```python
from build123d import *

# Parameters (mm, degrees)
SKETCH101_W          = 122
SKETCH101_H          = 70.3
SKETCH101_R          = 1.75
SKETCH101_R_2        = 1.55
SKETCH101_W_2        = 52.2
SKETCH101_H_2        = 52.2
PAD033_DEPTH         = 4
FILLET008_R          = 2
SKETCH102_W          = 2
SKETCH102_H          = 2.1
POCKET051_DEPTH      = 35.151
POCKET051_DEPTH_BACK = 35.151
SKETCH103_R          = 3
POCKET039_DEPTH      = 2.001
SKETCH104_W          = 4.202
SKETCH104_H          = 4.8
PAD035_DEPTH         = 10
CHAMFER004_SIZE2     = 9.99
CHAMFER004_SIZE      = 1.99


with BuildPart() as part:
    # Sketch101 → Pad033 (new body)
    with BuildSketch(Plane.XY):
        with Locations((31, 0)):
            Rectangle(SKETCH101_W, SKETCH101_H)
        with Locations((0, 31.75)):
            Circle(SKETCH101_R, mode=Mode.SUBTRACT)
        with Locations((-14, 30.5)):
            Circle(SKETCH101_R_2, mode=Mode.SUBTRACT)
        with Locations((60, 31.75)):
            Circle(SKETCH101_R, mode=Mode.SUBTRACT)
        with Locations((46, 30.5)):
            Circle(SKETCH101_R_2, mode=Mode.SUBTRACT)
        with Locations((60, -31.75)):
            Circle(SKETCH101_R, mode=Mode.SUBTRACT)
        with Locations((0, -31.75)):
            Circle(SKETCH101_R, mode=Mode.SUBTRACT)
        Rectangle(SKETCH101_W_2, SKETCH101_H_2, mode=Mode.SUBTRACT)
        with Locations((60, 0)):
            Rectangle(SKETCH101_W_2, SKETCH101_H_2, mode=Mode.SUBTRACT)
    extrude(amount=PAD033_DEPTH)

    # Fillet008
    fillet008_edges = [part.edges().sort_by_distance(p)[0] for p in [
        (31, 35.15, 4),
        (31, -35.15, 4),
    ]]
    fillet(fillet008_edges, radius=FILLET008_R)

    # Sketch102 → Pocket051 (cut, two sides)
    with BuildSketch(Plane.XZ) as pocket051_sk:
        with Locations((-29, 2.95)):
            Rectangle(SKETCH102_W, SKETCH102_H)
        with Locations((91, 1.05)):
            Rectangle(SKETCH102_W, SKETCH102_H)
    extrude(amount=-POCKET051_DEPTH, mode=Mode.SUBTRACT)
    extrude(pocket051_sk.sketch, amount=POCKET051_DEPTH_BACK, mode=Mode.SUBTRACT)

    # Sketch103 → Pocket039 (cut, through all)
    with BuildSketch(Plane.XY.offset(2)):
        with Locations((0, 31.75)):
            Circle(SKETCH103_R)
        with Locations((60, 31.75)):
            Circle(SKETCH103_R)
        with Locations((60, -31.75)):
            Circle(SKETCH103_R)
        with Locations((0, -31.75)):
            Circle(SKETCH103_R)
    extrude(amount=POCKET039_DEPTH, mode=Mode.SUBTRACT)

    # Sketch104 → Pad035 (join)
    with BuildSketch(Plane.XY):
        with Locations((-25.899, 30.75)):
            Rectangle(SKETCH104_W, SKETCH104_H)
        with Locations((-25.899, -30.75)):
            Rectangle(SKETCH104_W, SKETCH104_H)
    extrude(amount=-PAD035_DEPTH)

    # Chamfer004
    chamfer004_edges = [part.edges().sort_by_distance(p)[0] for p in [
        (-28, -30.75, 0),
        (-28, 30.75, 0),
    ]]
    chamfer004_side = part.faces().sort_by_distance((30.852667, -0.159179, 0))[0]
    chamfer(chamfer004_edges, length=CHAMFER004_SIZE, length2=CHAMFER004_SIZE2, reference=chamfer004_side)


solid = part.part
```
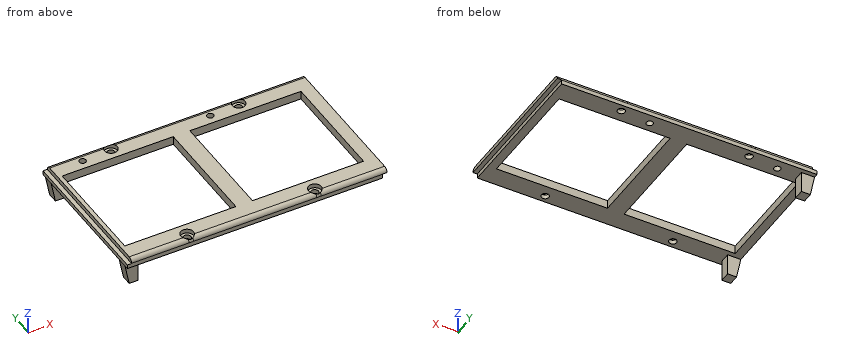
Input: part model. Units: mm. Frame: model coordinates. Round coordinates to 2 decimals unless told otherwise and drop trailing zeros. Loops run counter-clockwise (first coordinate to the right, second up) from the corner with the lowest first, then second, coordinate; pieces in that order, holes last. Notation, with made-up numbers: (53.25, 37.5) - (79.25, 37.5) arc R12 cw to (79.25, 60.5) - close; hole circle Ø6 at (39, -7). An arc over 180 degrees is marked (long way). One line per item, written item: value. Start each with the question number.
(1) Contact query for flat-ended pins moving along their axis: P1, Ø6.5, axis at x = 1, y = 33, coming from the +Z side; P2, Ø0.6, axis at x = 91, y = 9.5, coming from the -Z side; P3, Ø1.7, axis at y = -0.5, z = 3, coming from the -X side; P4, Ø3, axis at x = 61, y = 31, coming from the +Z side. Output: stop coordinate, or through.
(2) Section B-B, the plane y = 12.5. Return loops of the section in (x, z), plus the area to 3 significant figures.
(3) Section D-D, the plane y = -31.75. Count the separate pieces of the cut face and the enclosed holes in it, plus the area to 3 significant figures.
(4) Section C-C, the plane z = -7.5. Return loops of the section in (x, y).
(5) Section A-A, the plane x = -6. Return loops of the section in (y, z).
(6) Ray query, line 1 (X direction, y = -31.75, z = 1); line 2 (X direction, y = -31.75, z = 2.6); line 3 (Y direction, x = 0, z = 0.8). Return the intervals inside material, ascending. Write a range as [from, to].
Results below:
1. P1: z = 4
1. P2: z = 2.1
1. P3: x = -28
1. P4: z = 2
2. outline: (-30, 0) - (-26.1, 0) - (-26.1, 4) - (-28, 4) - (-28, 1.9) - (-30, 1.9) - close; (26.1, 0) - (33.9, 0) - (33.9, 4) - (26.1, 4) - close; (86.1, 0) - (90, 0) - (90, 2.1) - (92, 2.1) - (92, 4) - (86.1, 4) - close
2. area: 62.0 mm^2
3. separate pieces: 3
3. enclosed holes: 0
3. area: 494 mm^2
4. outline: (-28.5, -33.15) - (-23.8, -33.15) - (-23.8, -28.35) - (-28.5, -28.35) - close; (-28.5, 28.35) - (-23.8, 28.35) - (-23.8, 33.15) - (-28.5, 33.15) - close
5. outline: (-35.15, 0) - (-26.1, 0) - (-26.1, 4) - (-33.15, 4) arc R2 ccw to (-35.15, 2) - close; (26.1, 0) - (35.15, 0) - (35.15, 2) arc R2 ccw to (33.15, 4) - (26.1, 4) - close
6. line 1: [-30, -1.75], [1.75, 58.25], [61.75, 90]
6. line 2: [-28, -3], [3, 57], [63, 92]
6. line 3: [-35.15, -33.5], [-30, -26.1], [26.1, 30], [33.5, 35.15]
